from build123d import *

# Parameters (mm, degrees)
F1_DEPTH = 25.4
F2_T     = -2.54


with BuildPart() as f1:
    # F0 (on Top) → F1 (new body)
    with BuildSketch(Plane.XY):
        Polygon((-40.0050021708, 46.4459620416), (-49.4021475315, 46.4459620416), (-49.4021475315, 5.3670029156), (-93.434497714, -3.7616554182), (-73.2977539301, -23.3614202589), (-49.4021475315, -37.322897464), (-49.4021475315, -75.4484683275), (-19.0627854317, -75.4484683275), (-19.0627854317, -40.0077961385), (12.6190278679, -42.4242056906), (12.6190278679, -75.4484683275), (45.9117777646, -75.4484683275), (45.9117777646, -43.4981659055), (68.1964457035, -43.4981659055), (82.6948955655, -31.9531001151), (82.6948955655, -15.5752124265), (75.7141634822, 0), (67.9279565811, 46.4459620416), (49.6706403792, 46.4459620416), (71.9553008676, -23.6299112439), (25.7750339806, -18.2601120323), (-9.6656382084, 0), (-9.6656382084, 46.4459620416), (-19.0627854317, 46.4459620416), (-19.0627854317, 0), (-40.0050021708, 0), align=None)
    extrude(amount=F1_DEPTH)

    # F2
    f2_openings = [f1.faces().sort_by_distance(p)[0] for p in [
        (-1.371723, -22.717213, 25.4),
    ]]
    offset(amount=F2_T, openings=f2_openings, kind=Kind.INTERSECTION)


solid = f1.part
Verification items for the finished model (mm, model axes). A direction names the side the tool comes from. Give positions to 0.01 mm unless a question says otherwise; leave off trailing zeros. Write each loop counter-clockwise with the first axis right and the second up, starting at its lowest first coordinate (ties: lowest second). Pieces come first, ordered by that corner, then holes.
(1) Mould release check, pull along Y, two halves, no side actions. Record for faces 5 (the face through (-29, -2.54, 14)), 6 (the face through (-71.11, 0.867, 12.522)), 7 (the face through (57, -43.498, 13)): +Y half, -Y half, draft (parallel to the pull), parting line (faces both ways), or undercut.
(2) Cross-section at C-C (x = -37). Enter the section's corners in (y, z).
(3) Cross-section at A-A (y = -63). Enter the section's corners in (x, z).
(4) Cross-section at B-B (x = 63). Enter the section's corners in (y, z), plus the area to 3 significant figures.
(5) Cross-section at D-D (y = 23). Enter the section's corners in (x, z) (3 decimals), plus the area to 3 significant figures.
(6) Gauge pin test, flat ends, axial feed: pin 1 (10 mm diameter, centred on x = 35, z = 10.5, fed in from +Y); pin 2 (4.5 mm diameter, centred on y = -23, z = 15, fed in from -X); pin 3 (1 mm diameter, centred on x = 19, z = 16, fed in from +Y). Record the tip position at first contact, or that the pin passes through.
(7) Access from +Z, -Z, +X, -X, +Y, -Y to the whole of each face (thin tool, end or side, straight path). Record for faces 1 (the face through (-49.402, 26, 13)), 2 (the face through (71.876, 22.898, 12.522)), 3 (the face through (-14, 43.906, 14)), 4 (the face through (-29, 0, 13)).
(8) Material ranges on line 1 (X direction, y = -52, z = 14.75); line 2 (X direction, y = 25, z = 2.75) (3 decimals); line 3 (X direction, y = 40, z = 13.75) (1 decimal), recorded low to high.
Worked out:
1. face 5: undercut
1. face 6: +Y half
1. face 7: -Y half
2. outline: (-75.45, 0) - (0, 0) - (0, 25.4) - (-2.54, 25.4) - (-2.54, 2.54) - (-72.91, 2.54) - (-72.91, 25.4) - (-75.45, 25.4) - close
3. outline: (-49.4, 0) - (-19.06, 0) - (-19.06, 25.4) - (-21.6, 25.4) - (-21.6, 2.54) - (-46.86, 2.54) - (-46.86, 25.4) - (-49.4, 25.4) - close; (12.62, 0) - (45.91, 0) - (45.91, 25.4) - (43.37, 25.4) - (43.37, 2.54) - (15.16, 2.54) - (15.16, 25.4) - (12.62, 25.4) - close
4. outline: (-43.5, 0) - (-22.59, 0) - (-22.59, 25.4) - (-25.15, 25.4) - (-25.15, 2.54) - (-40.96, 2.54) - (-40.96, 25.4) - (-43.5, 25.4) - close; (4.53, 0) - (46.45, 0) - (46.45, 25.4) - (43.91, 25.4) - (43.91, 2.54) - (12.91, 2.54) - (12.91, 25.4) - (4.53, 25.4) - close
4. area: 526 mm2
5. outline: (-49.402, 0) - (-40.005, 0) - (-40.005, 25.4) - (-42.545, 25.4) - (-42.545, 2.54) - (-46.862, 2.54) - (-46.862, 25.4) - (-49.402, 25.4) - close; (-19.063, 0) - (-9.666, 0) - (-9.666, 25.4) - (-12.206, 25.4) - (-12.206, 2.54) - (-16.523, 2.54) - (-16.523, 25.4) - (-19.063, 25.4) - close; (57.127, 0) - (71.858, 0) - (71.858, 25.4) - (69.283, 25.4) - (69.283, 2.54) - (59.792, 2.54) - (59.792, 25.4) - (57.127, 25.4) - close
5. area: 437 mm2
6. pin 1: stops at y = -18.75
6. pin 2: stops at x = -75.98
6. pin 3: stops at y = -14.51
7. face 1: +Z, -Z, -X, +Y
7. face 2: +Z, -Z, +X, +Y
7. face 3: +Z
7. face 4: +Z, -Z, +Y
8. line 1: x = -49.4 to -46.86, -21.6 to -19.06, 12.62 to 15.16, 43.37 to 45.91
8. line 2: x = -49.402 to -46.862, -42.545 to -40.005, -19.063 to -16.523, -12.206 to -9.666, 56.491 to 59.156, 68.948 to 71.523
8. line 3: x = -49.4 to -46.9, -42.5 to -40, -19.1 to -16.5, -12.2 to -9.7, 51.7 to 54.4, 66.4 to 69
